from build123d import *

# Parameters (mm, degrees)
BOSS_EXTRUDE1_DEPTH = 3.048
SKETCH2_W           = 4.572
SKETCH2_H           = 5.08
SKETCH2_W_2         = 5.08
SKETCH2_H_2         = 2.54
SKETCH2_W_3         = 2.54
SKETCH2_H_3         = 4.572
SKETCH2_R           = 2.54
CUT_EXTRUDE1_DEPTH  = 3.048
SKETCH3_W           = 12.7
SKETCH3_H           = 3.048
SKETCH3_W_2         = 44.704
SKETCH3_H_2         = 12.7
BOSS_EXTRUDE2_DEPTH = 3.048
BOSS_EXTRUDE3_START = -3.048
SKETCH4_R           = 2.54
BOSS_EXTRUDE3_DEPTH = 3.048
SKETCH5_R           = 2.54
SKETCH5_W           = 5.08
SKETCH5_H           = 2.54
SKETCH5_W_2         = 4.572
SKETCH5_H_2         = 5.08
SKETCH5_W_3         = 2.54
SKETCH5_W_4         = 43.942
CUT_EXTRUDE2_DEPTH  = 114.63313911


with BuildPart() as part:
    # Sketch1 → Boss-Extrude1 (new body)
    with BuildSketch(Plane(origin=(0, 0, 0), x_dir=(1, 0, 0), z_dir=(0, 1, 0))):
        Polygon((0, 19.05), (0, 0), (19.05, 0), (19.05, 3.048), (31.75, 3.048), (31.75, 0), (47.752, 0), (47.752, 19.05), (50.8, 19.05), (50.8, 31.75), (47.752, 31.75), (47.752, 47.752), (31.75, 47.752), (31.75, 50.8), (19.05, 50.8), (19.05, 47.752), (0, 47.752), (0, 31.75), (3.048, 31.75), (3.048, 19.05), align=None)
    extrude(amount=BOSS_EXTRUDE1_DEPTH)

    # Sketch2 → Cut-Extrude1 (cut)
    with BuildSketch(Plane(origin=(0, 3.048, 0), x_dir=(1, 0, 0), z_dir=(0, 1, 0))):
        with Locations((5.334, 25.4)):
            Rectangle(SKETCH2_W, SKETCH2_H)
        with Locations((10.16, 25.4)):
            Rectangle(SKETCH2_W_2, SKETCH2_H)
        with Locations((10.16, 29.21)):
            Rectangle(SKETCH2_W_2, SKETCH2_H_2)
        with Locations((13.97, 25.4)):
            Rectangle(SKETCH2_W_3, SKETCH2_H)
        with Locations((10.16, 21.59)):
            Rectangle(SKETCH2_W_2, SKETCH2_H_2)
        with Locations((25.4, 13.97)):
            Rectangle(SKETCH2_W_2, SKETCH2_H_2)
        with Locations((25.4, 10.16)):
            Rectangle(SKETCH2_W_2, SKETCH2_H)
        with Locations((29.21, 10.16)):
            Rectangle(SKETCH2_W_3, SKETCH2_H)
        with Locations((21.59, 10.16)):
            Rectangle(SKETCH2_W_3, SKETCH2_H)
        with Locations((25.4, 5.334)):
            Rectangle(SKETCH2_W_2, SKETCH2_H_3)
        with Locations(Location((46.99, 25.4, 0), (0, 0, 270))):
            Circle(SKETCH2_R)
        with Locations(Location((25.4, 46.99, 0), (0, 0, 270))):
            Circle(SKETCH2_R)
    extrude(amount=-CUT_EXTRUDE1_DEPTH, mode=Mode.SUBTRACT)

    # Sketch3 → Boss-Extrude2 (add)
    with BuildSketch(Plane(origin=(0, 3.048, 0), x_dir=(1, 0, 0), z_dir=(0, 1, 0))):
        with Locations((25.4, 100.076)):
            Rectangle(SKETCH3_W, SKETCH3_H)
        Polygon((3.048, 82.55), (47.752, 82.55), (47.752, 98.552), (31.75, 98.552), (19.05, 98.552), (0, 98.552), (0, 82.55), align=None)
        with Locations((25.4, 76.2)):
            Rectangle(SKETCH3_W_2, SKETCH3_H_2)
        Polygon((0, 69.85), (0, 47.752), (19.05, 47.752), (19.05, 50.8), (31.75, 50.8), (31.75, 47.752), (47.752, 47.752), (47.752, 69.85), (3.048, 69.85), align=None)
    extrude(amount=-BOSS_EXTRUDE2_DEPTH)

    # Sketch4 → Boss-Extrude3 (add)
    with BuildSketch(Plane(origin=(0, 0, 0), x_dir=(-1, 0, 0), z_dir=(0, -1, 0)).offset(BOSS_EXTRUDE3_START)):
        with Locations((-25.4, 46.99)):
            Circle(SKETCH4_R)
    extrude(amount=BOSS_EXTRUDE3_DEPTH)

    # Sketch5 → Cut-Extrude2 (cut, through all)
    with BuildSketch(Plane(origin=(0, 3.048, 0), x_dir=(1, 0, 0), z_dir=(0, 1, 0))):
        with Locations(Location((25.4, 97.79, 0), (0, 0, 270))):
            Circle(SKETCH5_R)
        with Locations((10.16, 80.01)):
            Rectangle(SKETCH5_W, SKETCH5_H)
        with Locations((5.334, 76.2)):
            Rectangle(SKETCH5_W_2, SKETCH5_H_2)
        with Locations((10.16, 76.2)):
            Rectangle(SKETCH5_W, SKETCH5_H_2)
        with Locations((13.97, 76.2)):
            Rectangle(SKETCH5_W_3, SKETCH5_H_2)
        with Locations((10.16, 72.39)):
            Rectangle(SKETCH5_W, SKETCH5_H)
        with Locations((25.781, 66.04)):
            Rectangle(SKETCH5_W_4, SKETCH5_H)
        with Locations((21.971, 60.96)):
            Rectangle(SKETCH5_W_4, SKETCH5_H)
        with Locations((25.781, 55.88)):
            Rectangle(SKETCH5_W_4, SKETCH5_H)
        with Locations((21.971, 50.8)):
            Rectangle(SKETCH5_W_4, SKETCH5_H)
        with Locations((25.781, 45.72)):
            Rectangle(SKETCH5_W_4, SKETCH5_H)
        with Locations((21.971, 40.64)):
            Rectangle(SKETCH5_W_4, SKETCH5_H)
        with Locations((25.781, 35.56)):
            Rectangle(SKETCH5_W_4, SKETCH5_H)
    extrude(amount=-CUT_EXTRUDE2_DEPTH, mode=Mode.SUBTRACT)


solid = part.part
Check sheet for the modelled part. Datum: model origin and axes. Units: mm. A direction names the side the tool comes from. Round coordinates to 2 decimals unless told otherwise and drop trailing zeros. Order: outer loops, then holes, each group sorted by start corner. A loop starts at its lowest first (then second) coordinate and runs counter-clockwise, first axis right, second up.
(1) Go/stop test with flat-tipped pins: P1, Ø1.5, axis at x = 20.5, y = 1, coming from the +Z side; P2, Ø1.3, axis at x = 14.5, y = 1, coming from the -Z side; P3, Ø0.9, axis at y = 1, z = -100.5, coming from the -X side. Record where each tip stops, or that it passes through.
(2) Draft check along Z on faces 6 (the flat face through (50.8, 2, -25)), 7 (the flat face through (30, 2, -3.048)), 8 (the flat face through (7.62, 2, -22)). Enter one of: pulls with the +Z half, pulls with the -Z half, needs draft (parallel to the pull), parting line crosses it, or undercut.
(3) Access from +Z, -Z, +X, -X, +Y, -Y to the whole of each face (thin tool, end or side, straight path). Record for faces 1 (the flat face through (25, 2, -15.24)), 2 (the flat face through (30.48, 2, -10)), 3 (the flat face through (3.81, 2, -66)), 4 (the flat face through (47.752, 2, -41)), 5 (the flat face through (14, 2, -22.86)).
(4) Cross-section at A-A, the plane x = 17.5. State how many separate pieces and enclosed holes the cut face has, and give its area (3 significant figures).
(5) Scan lines: probe 1 along Z at (x, y) = (3, 1.7); probe 2 along X at (y, z) = (0.6, -25.4); probe 3 along X at (y, z) = (1.55, -97.79). Record each from-to range of solid material in increasing order.
(6) Cross-section at C-C, the plane x = 45.5. Enter the section's corners in (y, z).
(7) Cross-section at B-B, the plane z = -25.4. Enter the section's corners in (x, y), and give its area (3 significant figures).
Check sheet entries:
1. P1: stops at z = -3.05
1. P2: stops at z = -98.55
1. P3: stops at x = 19.05
2. face 6: needs draft
2. face 7: pulls with the +Z half
2. face 8: undercut
3. face 1: +Z, +Y, -Y
3. face 2: +Y, -Y
3. face 3: +X, +Y, -Y
3. face 4: -Z, +X, +Y, -Y
3. face 5: -X, +Y, -Y
4. separate pieces: 8
4. enclosed holes: 0
4. area: 246 mm2
5. probe 1: z = -98.55 to -82.55, -69.85 to -62.23, -59.69 to -52.07, -49.53 to -41.91, -39.37 to -31.75, -19.05 to 0
5. probe 2: x = 15.24 to 44.45, 49.53 to 50.8
5. probe 3: x = 0 to 22.86, 27.94 to 47.75
6. outline: (0, -98.55) - (3.05, -98.55) - (3.05, -67.31) - (0, -67.31) - close; (0, -64.77) - (3.05, -64.77) - (3.05, -57.15) - (0, -57.15) - close; (0, -54.61) - (3.05, -54.61) - (3.05, -46.99) - (0, -46.99) - close; (0, -44.45) - (3.05, -44.45) - (3.05, -36.83) - (0, -36.83) - close; (0, -34.29) - (3.05, -34.29) - (3.05, -27.46) - (0, -27.46) - close; (0, -23.34) - (3.05, -23.34) - (3.05, 0) - (0, 0) - close
7. outline: (15.24, 0) - (44.45, 0) - (44.45, 3.05) - (15.24, 3.05) - close; (49.53, 0) - (50.8, 0) - (50.8, 3.05) - (49.53, 3.05) - close
7. area: 92.9 mm2
